from build123d import *

# Parameters (mm, degrees)
PAD002_DEPTH    = 3
SKETCH004_R     = 1.5
PAD004_DEPTH    = 2.6
SKETCH005_W     = 10.2
SKETCH005_H     = 10.2
POCKET001_DEPTH = 2.5


with BuildPart() as part:
    # Sketch002 → Pad002 (new body)
    with BuildSketch(Plane.XY):
        Polygon((-5.369358, 9.3), (-10.738715, 0), (-5.369358, -9.3), (5.369358, -9.3), (10.738715, 0), (5.369358, 9.3), align=None)
    extrude(amount=PAD002_DEPTH)


with BuildPart() as part_1:
    # Body002 placement: moved
    add(part.part.moved(Location((0, 0, 3))))


with BuildPart() as part_2:
    # Clone placement: moved
    add(part_1.part.moved(Location((0, 0, -3))))

    # Sketch004 (on DatumPlane) → Pad004 (new body)
    with BuildSketch(Plane.XY.offset(3)):
        with Locations((-7.6, 0)):
            Circle(SKETCH004_R)
        with Locations((7.6, 0)):
            Circle(SKETCH004_R)
        with BuildLine():
            ThreePointArc((-3.5, 8.1), (-4.5, 7.1), (-3.5, 6.1))
            Line((-3.5, 6.1), (3.5, 6.1))
            ThreePointArc((3.5, 6.1), (4.5, 7.1), (3.5, 8.1))
            Line((3.5, 8.1), (-3.5, 8.1))
        make_face()
    extrude(amount=PAD004_DEPTH)

    # Sketch005 (on DatumPlane) → Pocket001 (cut)
    with BuildSketch(Plane.XY.offset(3)):
        Rectangle(SKETCH005_W, SKETCH005_H)
    extrude(amount=-POCKET001_DEPTH, mode=Mode.SUBTRACT)


solid = part_2.part
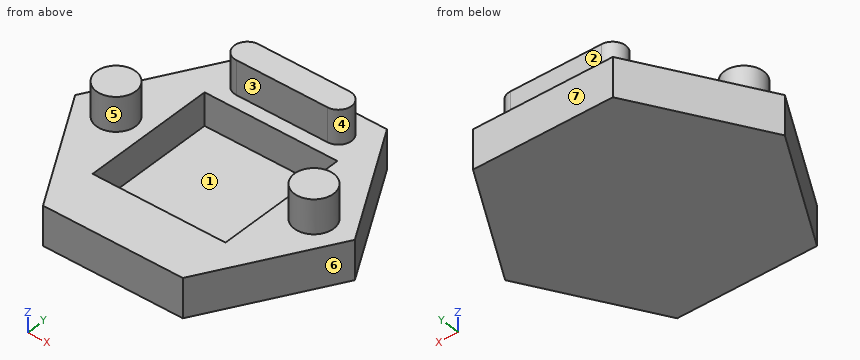
Geometry: final body of the model. Coordinates: model frame, mm. Face numbers are marked on the shaded views. A direction names the side the tool comes from. Give positions to 0.01 mm unless a question says otherwise; leave off trailing zeros. Loops run counter-clockwise (first coordinate to the right, second up) from the corner with the lowest first, then second, coordinate; pieces in that order, holes last. Notation, with made-up numbers: M 3.5,-36 L 8.5,-36 A13 cw 8.5,-28 Z; hole C 73,44.25 d7. An arc over 180 degrees is marked long. Put each result on its own line as item: value. Start each with the question number.
1) Cut plane D-D (y = 3). Output: boundary loops of the cut face in (x, z), then the cut area to 3 significant figures.
2) Cut plane B-B (x = -2). Output: boundary loops of the cut face in (y, z).
3) Pull-direction query (X, two-part tool) for the marked faces 5, 6 and 7; classes: pulls with the +X half, pulls with the -X half, needs draft (parallel to the pull), parting line crosses it, or undercut.
4) Contact query for flat-ended pins moving along their axis: pin 1 (6 mm diameter, centred on x = 3, y = -4, fed in from -Z); pin 2 (3 mm diameter, centred on x = -5, z = 5, fed in from +Y); pin 3 (3 mm diameter, centred on y = -2, z = 1.5, fed in from -X); pin 4 (1.3 mm diameter, centred on x = 0.5, z = 4.5, fed in from -Y). Output: stop coordinate, or through.
5) Cut plane A-A (z = 1.5). Output: boundary loops of the cut face in (x, y), then the cut area to 3 significant figures.
6) Access query for the marked faces 1, 2, 3 and 4. Directions: +Z, -Z, +X, -X, +Y, -Y. A direction counts if a zero-diameter tool reaches every point of the face in a straight line with its end or side. Return the directions, or none.
7) Ray query, line 1 along Y through (x, z) = (-3.5, 1.8); line 2 along X through (y, z) = (-2.5, 0.45); line 3 along X through (y, z) = (4.75, 2.7). Return the intervals inside material, ascending.
8) Cut plane C-C (z = 4). Output: boundary loops of the cut face in (x, y).
Verdict:
1. outline: M -9.01,0 L 9.01,0 L 9.01,3 L 5.1,3 L 5.1,0.5 L -5.1,0.5 L -5.1,3 L -9.01,3 Z
1. area: 28.5 mm2
2. outline: M -9.3,0 L 9.3,0 L 9.3,3 L 8.1,3 L 8.1,5.6 L 6.1,5.6 L 6.1,3 L 5.1,3 L 5.1,0.5 L -5.1,0.5 L -5.1,3 L -9.3,3 Z
3. face 5: undercut
3. face 6: pulls with the +X half
3. face 7: needs draft
4. pin 1: z = 0
4. pin 2: y = 8.1
4. pin 3: x = -10.45
4. pin 4: y = 6.1
5. outline: M -10.74,0 L -5.37,-9.3 L 5.37,-9.3 L 10.74,0 L 5.37,9.3 L -5.37,9.3 Z; hole M -5.1,-5.1 L 5.1,-5.1 L 5.1,5.1 L -5.1,5.1 Z
5. area: 196 mm2
6. face 1: +Z
6. face 2: +Z, +X, -X, +Y
6. face 3: +Z, +X, -X, -Y
6. face 4: +Z, +X
7. line 1: -9.3 to -5.1, 5.1 to 9.3
7. line 2: -9.3 to 9.3
7. line 3: -8 to -5.1, 5.1 to 8
8. outline: C -7.6,0 d3; M -3.5,6.1 L 3.5,6.1 A1 ccw 3.5,8.1 L -3.5,8.1 A1 ccw Z; C 7.6,0 d3
